Autodesk Inventor part; units mm, degrees
ref_plane "YZ Plane" through (0, 0, 0) normal (1, 0, 0) x (0, 1, 0)
ref_plane "XZ Plane" through (0, 0, 0) normal (0, 1, 0) x (-1, 0, 0)
ref_plane "XY Plane" through (0, 0, 0) normal (0, 0, 1) x (1, 0, 0)
sketch "Sketch1" plane through (0, 0, 0) normal (0, 0, 1) x (1, 0, 0)
  line L0 (0, 0) -> (0, 152.4)
  line L1 (0, 0) -> (365.76, 0)
  line L2 (365.76, 0) -> (365.76, 76.2)
  line L3 (365.76, 76.2) -> (0, 152.4)
  line L4 (3.048, 0) -> (6.929, 0)
  dimension "d0" = 152.4
  dimension "d1" = 365.76
extrude "Extrusion1" add sketch "Sketch1" along normal blind 457.2
sketch "Sketch2" plane through (0, 0, 0) normal (0, -1, 0) x (1, 0, 0)
  line L0 (11.3168, 439.6936) -> (353.778, 439.6936)
  line L1 (353.778, 439.6936) -> (353.778, 12.302)
  line L2 (353.778, 12.302) -> (11.3168, 12.302)
  line L3 (11.3168, 12.302) -> (11.3168, 439.6936)
  point P0 (0, 0)
extrude "Extrusion2" cut sketch "Sketch2" against normal blind 426.72
sketch "Sketch3" plane through (0, 0, 457.2) normal (0, 0, 1) x (1, 0, 0)
  line L0 (0, 0) -> (365.76, 0)
  line L1 (0, 0) -> (365.76, 0)
  line L2 (365.76, 0) -> (365.76, -3.048)
  line L3 (365.76, -3.048) -> (0, -3.048)
  line L4 (0, -3.048) -> (0, 0)
  dimension "d6" = 3.048
extrude "Extrusion3" add sketch "Sketch3" against normal blind 457.2
sketch "Sketch4" plane through (365.76, 76.2, 457.2) normal (1, 0, 0) x (0, 0, -1)
  point P0 (457.2, -76.2)
sketch "Sketch5" plane through (365.76, 76.2, 457.2) normal (1, 0, 0) x (0, 0, -1)
  line L0 (0, -79.248) -> (0, 0)
  line L1 (457.2, 0) -> (457.2, -79.248)
  line L2 (457.2, 0) -> (457.2, 76.2)
  line L3 (457.2, 0) -> (441.96, 0)
  line L4 (457.2, 0) -> (0, 0)
  line L5 (17.5064, -76.2) -> (444.898, -76.2)
  line L6 (441.96, 0) -> (228.6, 0)
  line L7 (228.6, 0) -> (228.6, -76.2)
  line L8 (228.6, -76.2) -> (441.96, -76.2)
  line L9 (441.96, -76.2) -> (441.96, 0)
  point P0 (457.2, -76.2)
  dimension "d24" = 15.24
  dimension "d25" = 213.36
extrude "Extrusion4" [suppressed]
sketch "Sketch6" plane through (365.76, -3.048, 457.2) normal (1, 0, 0) x (0, 0, -1)
  point P0 (457.2, 3.048)
sketch "Sketch7" plane through (11.3168, 0, 12.302) normal (0, 1, 0) x (1, 0, 0)
  circle A0 centre (73.0445, -381.6111) radius 13.6067
  circle A1 centre (136.9959, -61.8544) radius 12.9084
  point P0 (-11.3168, 12.302)
extrude "Extrusion5" add sketch "Sketch7" along normal blind 274.32
sketch "Sketch8" plane through (0, 0, 457.2) normal (0, 0, 1) x (1, 0, 0)
  point P0 (0, 0)
sketch "Sketch9" plane through (11.3168, 0, 12.302) normal (0, 1, 0) x (1, 0, 0)
  line L0 (354.4432, -444.898) -> (-11.3168, -444.898)
  line L1 (-11.3168, -444.898) -> (342.4612, -444.898)
  line L2 (342.4612, -444.898) -> (342.4612, -427.3916)
  line L3 (342.4612, -427.3916) -> (-11.3168, -427.3916)
  line L4 (-11.3168, -427.3916) -> (-11.3168, -444.898)
  point P0 (-11.3168, 12.302)
extrude "Extrusion6" add sketch "Sketch9" along normal blind 396.24
sketch "Sketch10" plane through (0, 0, 457.2) normal (0, 0, 1) x (1, 0, 0)
  line L0 (0, 396.24) -> (0, -3.048)
  line L1 (353.778, 396.24) -> (0, 396.24)
  line L2 (0, 396.24) -> (353.778, 396.24)
  line L3 (353.778, 78.6962) -> (353.778, 396.24)
  line L4 (353.778, 396.24) -> (353.778, 320.04)
  line L5 (353.778, 320.04) -> (0, 396.24)
  point P0 (0, 0)
  dimension "d17" = 76.2
extrude "Extrusion7" cut sketch "Sketch10" against normal blind 3048
sketch "Sketch11" plane through (11.3168, 0, 12.302) normal (0, 1, 0) x (1, 0, 0)
  line L0 (-11.3168, -444.898) -> (-11.3168, 12.302)
  line L1 (354.4432, -444.898) -> (354.4432, 12.302)
  line L2 (-11.3168, -0.0453) -> (354.4432, -0.0453)
  line L3 (354.4432, -0.0453) -> (354.4432, 12.302)
  line L4 (354.4432, 12.302) -> (-11.3168, 12.302)
  line L5 (-11.3168, 12.302) -> (-11.3168, -0.0453)
  point P0 (354.4432, -109.618)
extrude "Extrusion8" add sketch "Sketch11" along normal blind 396.24
sketch "Sketch12" plane through (11.3168, 0, 12.3473) normal (0, 0, 1) x (1, 0, 0)
  line L0 (354.4432, 396.24) -> (-11.3168, 396.24)
  line L1 (-11.3168, 396.24) -> (354.4432, 317.798)
  line L2 (354.4432, 396.24) -> (354.4432, -3.048)
  line L3 (-11.3168, 396.24) -> (342.4612, 320.04)
  line L4 (354.4432, 396.24) -> (-11.3168, 396.24)
  point P0 (-11.3168, 0)
extrude "Extrusion9" cut sketch "Sketch12" against normal blind 3048
sketch "Sketch13" plane through (353.778, 0, 439.6936) normal (0, 0, -1) x (-1, 0, 0)
  point P0 (353.778, 0)
sketch "Sketch14" plane through (353.778, 0, 439.6936) normal (0, 0, -1) x (-1, 0, 0)
  point P0 (353.778, 0)
sketch "Sketch15" plane through (365.76, -3.048, 457.2) normal (1, 0, 0) x (0, 0, -1)
  line L0 (444.8527, 79.248) -> (0, 79.248)
  line L1 (444.8527, 81.7442) -> (444.8527, 3.048)
  line L2 (17.5064, 3.048) -> (444.8527, 3.048)
  line L3 (444.8527, 70.104) -> (231.4927, 70.104)
  line L4 (231.4927, 70.104) -> (231.4927, 3.048)
  line L5 (231.4927, 3.048) -> (444.8527, 3.048)
  line L6 (444.8527, 3.048) -> (444.8527, 70.104)
  point P0 (457.2, 3.048)
  dimension "d26" = 9.144
  dimension "d27" = 213.36
extrude "Extrusion10" cut sketch "Sketch15" against normal blind 25.4
properties part number "new base part"
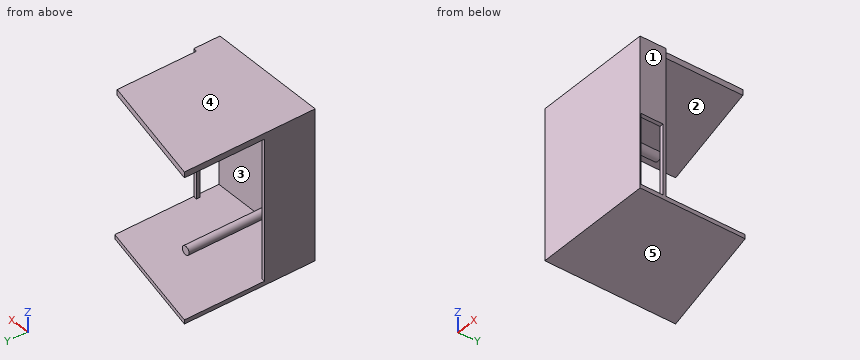
Can you work these out from the model? Positions are in its coordinate system, mm. Face numbers are marked on the shaded views. A direction names the side the tool comes from. Coordinates: 2 decimals unless noted, no trailing zeros. Loops run counter-clockwise (first coordinate to the right, second up) from the corner with the lowest first, then second, coordinate; pieces in that order, holes last.
1) Imagine slicing it at C-C on x = 86. List the corners of the cut face in (y, z) for me.
2) Imagine slicing it at B-B on y = 46. List the corners of the cut face in (x, z) for me.
3) I need wall thicknesses on probe 1 along X at (y, z) = (74, 52.5); probe 2 along Z at (x, y) = (66.5, 136.5); probe 3 along Y at (x, z) = (21, 182). Which ranges of each line are inside material? Lowest first, please.
4) Imagine slicing it at D-D on z = 260. List the corners of the cut face in (x, y) for me, plus the area to 3 significant figures.
5) For pin 1 (4 mm diameter, centred on x = 190, z = 268.5, fed in from +Y); pin 2 (8 mm diameter, centred on y = 115, z = 242.5, fed in from +X); pin 3 (8 mm diameter, centred on y = 247, z = 67.5, fed in from -X), each with a flat end and sliding along its axis, tell me the tip position at first contact or that it passes through.
6) Which directions (+Z, -Z, +X, -X, +Y, -Y) give clear straight access to the entire face, cutting with the end or side of a thin tool? Please do the marked faces 1 and 2.
7) Thinking about a two-plate mould opening in Z: for the marked faces 3, 4 and 5, which applies, pulls with the +Z half, pulls with the -Z half, needs draft (parallel to the pull), parting line crosses it, or undercut?
8) Imagine slicing it at A-A on z = 119. List the corners of the cut face in (x, y) for me, plus the area to 3 significant figures.
Completed:
1. outline: (-3.05, 0) - (377.8, 0) - (377.8, 12.35) - (0, 12.35) - (0, 380.41) - (274.32, 380.41) - (274.32, 407.42) - (0, 407.42) - (0, 439.69) - (377.72, 439.69) - (377.72, 457.2) - (-3.05, 457.2) - close
2. outline: (0, 0) - (365.76, 0) - (365.76, 12.35) - (11.32, 12.35) - (11.32, 439.69) - (353.78, 439.69) - (353.78, 225.71) - (365.76, 225.71) - (365.76, 457.2) - (0, 457.2) - close; circle Ø27.21 at (84.36, 393.91); circle Ø25.82 at (148.31, 74.16)
3. probe 1: x = 0 to 11.32, 353.78 to 365.76
3. probe 2: z = 0 to 12.35, 439.69 to 457.2
3. probe 3: y = -3.05 to 0
4. outline: (0, -3.05) - (365.76, -3.05) - (365.76, 76.2) - (353.78, 78.7) - (353.78, 0) - (11.32, 0) - (11.32, 150.04) - (0, 152.4) - close
4. area: 3,750 mm2
5. pin 1: stops at y = 0
5. pin 2: stops at x = 11.32
5. pin 3: stops at x = 135.68
6. face 1: +Z, -Z, +X, +Y, -Y
6. face 2: +Y
7. face 3: undercut
7. face 4: pulls with the +Z half
7. face 5: pulls with the -Z half
8. outline: (0, -3.05) - (365.76, -3.05) - (365.76, 0) - (11.32, 0) - (11.32, 150.04) - (0, 152.4) - close; (353.78, 67.06) - (365.76, 67.06) - (365.76, 76.2) - (353.78, 78.7) - close
8. area: 2,950 mm2
